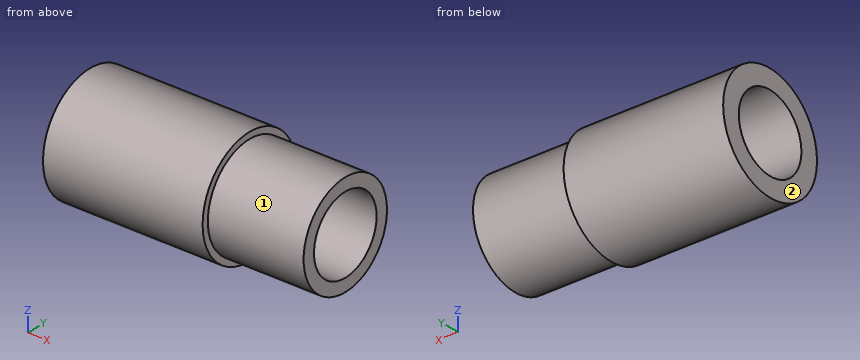
from build123d import *

# Parameters (mm, degrees)
F0_R          = 4
F0_R_2        = 3
F1_DEPTH      = 7.5
F1_DEPTH_BACK = 12.5
F0_R_3        = 4.5
F2_DEPTH      = 12.5


with BuildPart() as f1:
    # F0 (on Right) → F1 (new body, two sides)
    with BuildSketch(Plane.YZ) as f1_sk:
        Circle(F0_R)
        Circle(F0_R_2, mode=Mode.SUBTRACT)
    extrude(amount=F1_DEPTH)
    extrude(f1_sk.sketch, amount=-F1_DEPTH_BACK)

    # F0 (on Right) → F2 (join)
    with BuildSketch(Plane.YZ):
        Circle(F0_R_3)
        Circle(F0_R, mode=Mode.SUBTRACT)
    extrude(amount=-F2_DEPTH)


solid = f1.part
Geometry: final body of the model. Coordinates: model frame, mm. Face numbers are marked on the shaded views. A direction names the side the tool comes from. Give positions to 0.01 mm unless a question says otherwise; leave off trailing zeros. Order: outer loops, then holes, each group sorted by start corner. A loop starts at its lowest first (then second) coordinate and runs counter-clockwise, first axis right, second up. Notation, with made-up numbers: (87, 88.5) -> (127, 88.5) arc R29 ccw to (127, 118.5) -> close; hole circle Ø2 at (12, 73). An arc over 180 degrees is marked (long way). Answer as a JSON object with one key per item and string values.
Q1. Material intervals for probe 1 along Z at (x, y) = (5.25, 0); probe 2 along Z at (x, y) = (-9.5, 0); probe 3 along X at (y, z) = (-2.75, -3), sorted ascending.
Entries:
{"probe 1": "z = -4 to -3, 3 to 4", "probe 2": "z = -4.5 to -3, 3 to 4.5", "probe 3": "x = -12.5 to 0"}
Q2. Access query for the marked faces 1 and 2. Directions: +Z, -Z, +X, -X, +Y, -Y. A direction counts if a zero-diameter tool reaches every point of the face in a straight line with its end or side. Return the directions, or none.
Entries:
{"face 1": "+X", "face 2": "+Z, -Z, -X, +Y, -Y"}
Q3. Section B-B (z = -0.75). Output: boundary loops of the cut face in (x, y).
Entries:
{"outline": "(-12.5, -4.44) -> (0, -4.44) -> (0, -3.93) -> (7.5, -3.93) -> (7.5, -2.9) -> (-12.5, -2.9) -> close; (-12.5, 2.9) -> (7.5, 2.9) -> (7.5, 3.93) -> (0, 3.93) -> (0, 4.44) -> (-12.5, 4.44) -> close"}
Q4. Section A-A (y = 0). Output: boundary loops of the cut face in (x, z).
Entries:
{"outline": "(-12.5, -4.5) -> (0, -4.5) -> (0, -4) -> (7.5, -4) -> (7.5, -3) -> (-12.5, -3) -> close; (-12.5, 3) -> (7.5, 3) -> (7.5, 4) -> (0, 4) -> (0, 4.5) -> (-12.5, 4.5) -> close"}
Q5. Section D-D (x = 4.75). Output: boundary loops of the cut face in (y, z).
Entries:
{"outline": "circle Ø8 at (0, 0); hole circle Ø6 at (0, 0)"}
Q6. Section C-C (x = -2.25). Output: boundary loops of the cut face in (y, z).
Entries:
{"outline": "circle Ø9 at (0, 0); hole circle Ø6 at (0, 0)"}
Q7. First-contact query: pin 1 (3 mm diameter, centred on x = -2, z = 2, fed in from -Y); pin 2 (5 mm diameter, centred on y = 0, z = 0, fed in from -X); pin 3 (1.5 mm diameter, centred on x = 1, y = 3, fed in from -Z). Flat tips, straight axial feed; report the tip coordinate or a pass-through.
Entries:
{"pin 1": "stops at y = -4.47", "pin 2": "passes through", "pin 3": "stops at z = -3.31"}
